CAD build for the part. Positions are in the model's coordinates, mm. Face numbers are marked on the shaded views. A direction names the side the tool comes from. Coordinates: 2 decimals unless noted, no trailing zeros. Write each loop counter-clockwise with the first axis right and the second up, starting at its lowest first coordinate (ties: lowest second). Pieces come first, ordered by that corner, then holes. Notation, with made-up numbers: M -27.75,44 L 21.25,44 A17 ccw 21.25,71 Z; hole C 5.5,-24 d8. An arc over 180 degrees is marked long. Put each result on its own line as item: value. Start each with the question number.
```python
from build123d import *

# Parameters (mm, degrees)
SKETCH_1_R           = 17
EXTRUDE_1_DEPTH      = 34
EXTRUDE_START        = 6
SKETCH_2_R           = 40
EXTRUDE_2_DEPTH      = 12
SKETCH_3_R           = 27
EXTRUDE_3_DEPTH      = 6
SKETCH_4_R           = 24
SKETCH_4_R_2         = 12
CUT_EXTRUDE_1_DEPTH  = 9
SKETCH_5_OUTSIDE_W   = 105.628
SKETCH_5_OUTSIDE_H   = 105.628
SKETCH_5_OUTSIDE_W_2 = 58
SKETCH_5_OUTSIDE_H_2 = 80
SKETCH_5_OUTSIDE_R   = 8
CUT_EXTRUDE_2_DEPTH  = 35


with BuildPart() as part:
    # 草圖1 → 填料-伸長1 (new body)
    with BuildSketch(Plane.XY):
        Circle(SKETCH_1_R)
    extrude(amount=EXTRUDE_1_DEPTH)

    # 草圖2 → 填料-伸長2 (add)
    with BuildSketch(Plane.XY.offset(EXTRUDE_START)):
        Circle(SKETCH_2_R)
    extrude(amount=EXTRUDE_2_DEPTH)

    # 草圖3 → 填料-伸長3 (add)
    with BuildSketch(Plane(origin=(0, 0, 6), x_dir=(-1, 0, 0), z_dir=(0, 0, -1))):
        Circle(SKETCH_3_R)
    extrude(amount=EXTRUDE_3_DEPTH)

    # 草圖4 → 除料-伸長1 (cut)
    with BuildSketch(Plane(origin=(0, 0, 0), x_dir=(-1, 0, 0), z_dir=(0, 0, -1))):
        Circle(SKETCH_4_R)
        Circle(SKETCH_4_R_2, mode=Mode.SUBTRACT)
    extrude(amount=-CUT_EXTRUDE_1_DEPTH, mode=Mode.SUBTRACT)

    # 草圖5 outside → 除料-伸長2 (cut, through all)
    with BuildSketch(Plane(origin=(0, 0, 0), x_dir=(-1, 0, 0), z_dir=(0, 0, -1))):
        Rectangle(SKETCH_5_OUTSIDE_W, SKETCH_5_OUTSIDE_H)
        Rectangle(SKETCH_5_OUTSIDE_W_2, SKETCH_5_OUTSIDE_H_2, mode=Mode.SUBTRACT)
        Circle(SKETCH_5_OUTSIDE_R)
    extrude(amount=-CUT_EXTRUDE_2_DEPTH, mode=Mode.SUBTRACT)


solid = part.part
```
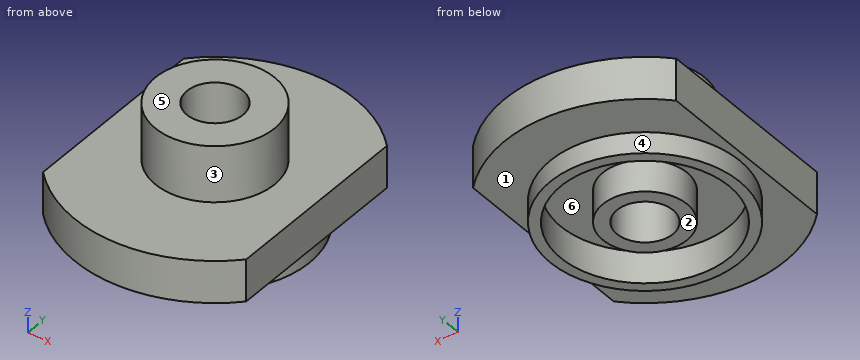
(1) Drop flat-ended pins along their axis: pin 1 (12 mm diameter, centred on y = 17.5, z = 27.5, fed in from -X); pin 2 (3 mm diameter, centred on x = 18, y = -28, fed in from -Z); pin 3 (3 mm diameter, centred on x = -0.5, z = 8, fed in from +Y). Give the stop position or say it passes through.
(2) Which spindle directions (+Z, -Z, +X, -X, +Y, -Y) get a long thin tool onto all of the face, cutting with end or side? Do the marked faces 1, 2 and 3. Say none if no direction does.
(3) Two-plate mould, pull along X, no slides. Class the marked faces 4, 5 and 6: +X half, -X half, draft (parallel to the pull), parting line (faces both ways), or undercut.
(4) Drill centre lines: line 1 (Y direction, x = 0, z = 2); line 2 (Y direction, x = 0, z = 25); line 3 (Z direction, x = 16.5, y = 22). Where is each one in solid material? Low to high. Write a range as [from, to].
(5) Slice it at D-D, the plane z = 17. Write the cut outline in (x, y), then the cut area to 3 significant figures.
(6) Slice it at C-C, the plane y = 0. Write the cut outline in (x, z), then the cut area to 3 significant figures.
(7) Slice it at B-B, the plane x = 0. Write the cut outline in (y, z).
(8) Slice it at A-A, the plane z = 7. Write the cut outline in (x, y), then the cut area to 3 significant figures.
Result set:
1. pin 1: stops at x = -12.52
1. pin 2: stops at z = 6
1. pin 3: stops at y = 40
2. face 1: -Z
2. face 2: -Z, +X, -X, +Y, -Y
2. face 3: +Z
3. face 4: parting line
3. face 5: draft
3. face 6: undercut
4. line 1: y = [-27, -24], [-12, -8], [8, 12], [24, 27]
4. line 2: y = [-17, -8], [8, 17]
4. line 3: z = [6, 18]
5. outline: M -29,-27.55 A40 ccw 29,-27.55 L 29,27.55 A40 ccw -29,27.55 Z; hole C 0,0 d16
5. area: 3,990 mm^2
6. outline: M -29,6 L -27,6 L -27,0 L -24,0 L -24,9 L -12,9 L -12,0 L -8,0 L -8,34 L -17,34 L -17,18 L -29,18 Z; M 8,0 L 12,0 L 12,9 L 24,9 L 24,0 L 27,0 L 27,6 L 29,6 L 29,18 L 17,18 L 17,34 L 8,34 Z
6. area: 804 mm^2
7. outline: M -40,6 L -27,6 L -27,0 L -24,0 L -24,9 L -12,9 L -12,0 L -8,0 L -8,34 L -17,34 L -17,18 L -40,18 Z; M 8,0 L 12,0 L 12,9 L 24,9 L 24,0 L 27,0 L 27,6 L 40,6 L 40,18 L 17,18 L 17,34 L 8,34 Z
8. outline: M -29,-27.55 A40 ccw 29,-27.55 L 29,27.55 A40 ccw -29,27.55 Z; C 0,0 d24; hole C 0,0 d48; hole C 0,0 d16
8. area: 2,630 mm^2
